Geometry check sheet. Reference: the model listing, model coordinates, mm. Face numbers are marked on the shaded views. A direction names the side the tool comes from. Give positions to 0.01 mm unless a question says otherwise; leave off trailing zeros. Order: outer loops, then holes, each group sorted by start corner. A loop starts at its lowest first (then second) coordinate and runs counter-clockwise, first axis right, second up. Notation, with made-up numbers: M 66,53 L 84,53 A16 ccw 84,61 Z; hole C -25.5,45.25 d8. An arc over 180 degrees is marked long. One line per question, with ' | ' between items. Start each with the question number.
from build123d import *

# Parameters (mm, degrees)
F0_R     = 8
F1_DEPTH = 9
F3_DEPTH = 9
F4_R     = 8
F5_DEPTH = 9
F7_DEPTH = 9
F8_R     = 8
F9_DEPTH = 9


# Not quite as in the source:
# - a pattern or mirror of a feature is missing from the dataset's text; its kind, count and spacing are read off the source's solid


with BuildPart() as f1:
    # F0 (on Top) → F1 (new body)
    with BuildSketch(Plane.XY):
        with BuildLine():
            ThreePointArc((17.3845397472, 29.3333333333), (17.7988188757, 31.316337087), (17.9876500843, 33.3333333333))
            ThreePointArc((17.9876500843, 33.3333333333), (0, 52), (-17.9876500843, 33.3333333333))
            ThreePointArc((-17.9876500843, 33.3333333333), (-20.5007344281, 26.7550020016), (-26.9814751265, 24))
            Line((-26.9814751265, 24), (-72, 24))
            Line((-72, 24), (-72, -24))
            Line((-72, -24), (-26.9814751265, -24))
            ThreePointArc((-26.9814751265, -24), (-20.5007344281, -26.7550020016), (-17.9876500843, -33.3333333333))
            ThreePointArc((-17.9876500843, -33.3333333333), (0, -52), (17.9876500843, -33.3333333333))
            ThreePointArc((17.9876500843, -33.3333333333), (17.7988188757, -31.316337087), (17.3845397472, -29.3333333333))
            ThreePointArc((17.3845397472, -29.3333333333), (18.9353811923, -21.5227744249), (26.0768096208, -18))
            Line((26.0768096208, -18), (38.5327786207, -18))
            Line((38.5327786207, -18), (38.5327786207, 18))
            Line((38.5327786207, 18), (26.0768096208, 18))
            ThreePointArc((26.0768096208, 18), (18.9353811923, 21.5227744249), (17.3845397472, 29.3333333333))
        make_face()
        with Locations((0, -34)):
            Circle(F0_R, mode=Mode.SUBTRACT)
        with Locations((0, 34)):
            Circle(F0_R, mode=Mode.SUBTRACT)
    extrude(amount=F1_DEPTH)

    # F2 (on face) → F3 (join)
    with BuildSketch(Plane.XZ.offset(24)):
        with BuildLine():
            Line((-36.0185248735, 18), (-36.0185248735, 30))
            ThreePointArc((-36.0185248735, 30), (-54.0264671065, 47.9999982478), (-72.0185178648, 29.9841155356))
            Line((-72.0185178648, 29.9841155356), (-72, 9))
            Line((-72, 9), (-27.0185248735, 9))
            ThreePointArc((-27.0185248735, 9), (-33.3824859042, 11.6360389693), (-36.0185248735, 18))
        make_face()
    f3 = extrude(amount=-F3_DEPTH)

    # F3_copies: F3 across plane
    add(f3.mirror(Plane.ZX))

    # F4 (on face) → F5 (cut, through all)
    with BuildSketch(Plane.XZ.offset(24)):
        with Locations((-54.0185248735, 30)):
            Circle(F4_R)
    f5 = extrude(amount=-F5_DEPTH, mode=Mode.SUBTRACT)

    # F5_copies: F5 across plane
    add(f5.mirror(Plane.ZX), mode=Mode.SUBTRACT)

    # F6 (on face) → F7 (join)
    with BuildSketch(Plane.YZ.offset(38.5327786207)):
        with BuildLine():
            Line((18, 9), (18, 30))
            ThreePointArc((18, 30), (0, 48), (-18, 30))
            Line((-18, 30), (-18, 9))
            Line((-18, 9), (18, 9))
        make_face()
    extrude(amount=-F7_DEPTH)

    # F8 (on face) → F9 (cut, through all)
    with BuildSketch(Plane.YZ.offset(38.5327786207)):
        with Locations((0, 30)):
            Circle(F8_R)
    extrude(amount=-F9_DEPTH, mode=Mode.SUBTRACT)


solid = f1.part
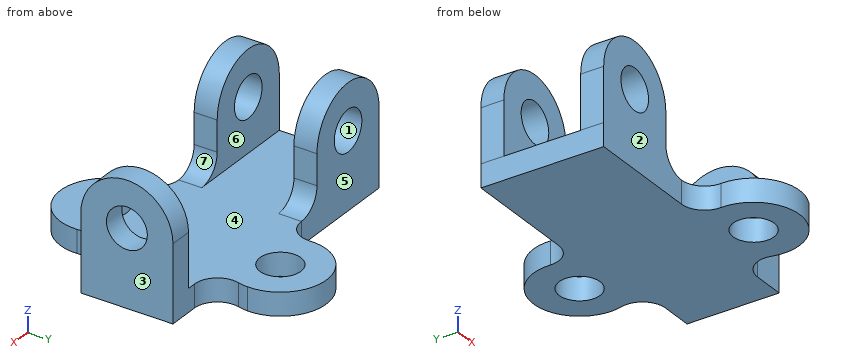
Item 1: Material ranges on line 1 along Y through (x, z) = (-45, 34); line 2 along Z through (x, y) = (13.5, -15); line 3 along Z through (x, y) = (36, 0), recorded low to high.
Item 2: Mould release check, pull along X, two halves, no side actions. Record for the marked faces 1, 2 and 3: released by +X, released by -X, zero draft, split by the parting line, or undercut.
Item 3: Set-up check for the marked faces 4, 5, 6 and 7: record each of +Z, -Z, +X, -X, +Y, -Y from which the full face is reachable in a straight line by a thin tool's end or side.
Item 4: Depth check by flat-ended pin: pin 1 (12 mm diameter, centred on y = 24.5, z = 9.5, fed in from -X); pin 2 (14.5 mm diameter, centred on x = -54.02, z = 30, fed in from -Y); pin 3 (18 mm diameter, centred on y = 5.5, z = 27, fed in from -X); pin 4 (6 mm diameter, centred on x = 35, z = 8, fed in from -Y). Enter the tip coordinate at first touch or a pass-through.
Item 5: Cross-section at B-B, the plane x = 0. Record the cut outline in (y, z), plus the area to 3 significant figures.
Item 6: Cross-section at C-C, the plane z = 32. Record the cut outline in (x, y), plus the area to 3 significant figures.
Item 7: Cross-section at A-A, the plane y = 0. Record the cut outline in (x, z).
Item 8: Cross-section at D-D, the plane z = 11.5. Record the cut outline in (x, y), plus the area to 3 significant figures.
Outcome:
1) line 1: y = -24 to -15, 15 to 24 | line 2: z = 0 to 9 | line 3: z = 0 to 22, 38 to 48
2) face 1: undercut | face 2: zero draft | face 3: released by +X
3) face 4: +Z | face 5: +Z, -Z, -X, +Y | face 6: +Z, -X | face 7: +Z, +Y, -Y
4) pin 1: stops at x = -72.01 | pin 2: passes through | pin 3: stops at x = 29.53 | pin 4: stops at y = -18
5) outline: M -52,0 L -42,0 L -42,9 L -52,9 Z; M -26,0 L 26,0 L 26,9 L -26,9 Z; M 42,0 L 52,0 L 52,9 L 42,9 Z | area: 648 mm²
6) outline: M -71.91,-24 L -61.76,-24 L -61.76,-15 L -71.91,-15 Z; M -71.91,15 L -61.76,15 L -61.76,24 L -71.91,24 Z; M -46.27,-24 L -36.13,-24 L -36.13,-15 L -46.27,-15 Z; M -46.27,15 L -36.13,15 L -36.13,24 L -46.27,24 Z; M 29.53,-17.89 L 38.53,-17.89 L 38.53,-7.75 L 29.53,-7.75 Z; M 29.53,7.75 L 38.53,7.75 L 38.53,17.89 L 29.53,17.89 Z | area: 548 mm²
7) outline: M -72,0 L 38.53,0 L 38.53,22 L 29.53,22 L 29.53,9 L -72,9 Z; M 29.53,38 L 38.53,38 L 38.53,48 L 29.53,48 Z
8) outline: M -72,-24 L -33.24,-24 L -33.24,-15 L -72,-15 Z; M -72,15 L -33.24,15 L -33.24,24 L -72,24 Z; M 29.53,-18 L 38.53,-18 L 38.53,18 L 29.53,18 Z | area: 1,020 mm²
